```python
from build123d import *

# Parameters (mm, degrees)
SKETCH1_W           = 1000
SKETCH1_H           = 141
SKETCH1_H_2         = 170
SKETCH1_H_3         = 32
BOSS_EXTRUDE1_DEPTH = 40
SKETCH2_W           = 44
SKETCH2_H           = 44
BOSS_EXTRUDE2_DEPTH = 296
SKETCH3_W           = 44
SKETCH3_H           = 40
BOSS_EXTRUDE3_DEPTH = 100
SKETCH4_W           = 44
SKETCH4_H           = 44
BOSS_EXTRUDE4_DEPTH = 209


with BuildPart() as part:
    # Sketch1 → Boss-Extrude1 (new body)
    with BuildSketch(Plane(origin=(0, 0, 0), x_dir=(1, 0, 0), z_dir=(0, 1, 0))):
        Polygon((-500, 236), (-500, 345), (-540, 345), (-540, -345), (-500, -345), (-500, -283), (500, -283), (500, -345), (540, -345), (540, 345), (500, 345), (500, 236), align=None)
        with Locations((0, -168.5)):
            Rectangle(SKETCH1_W, SKETCH1_H, mode=Mode.SUBTRACT)
        with Locations((0, 31)):
            Rectangle(SKETCH1_W, SKETCH1_H_2, mode=Mode.SUBTRACT)
        with Locations((0, 176)):
            Rectangle(SKETCH1_W, SKETCH1_H_3, mode=Mode.SUBTRACT)
    extrude(amount=BOSS_EXTRUDE1_DEPTH)

    # Sketch2 → Boss-Extrude2 (add)
    with BuildSketch(Plane(origin=(0, 40, 0), x_dir=(1, 0, 0), z_dir=(0, 1, 0))):
        with Locations((-123, 214)):
            Rectangle(SKETCH2_W, SKETCH2_H)
        with Locations((123, 214)):
            Rectangle(SKETCH2_W, SKETCH2_H)
        with Locations((-123, 138)):
            Rectangle(SKETCH2_W, SKETCH2_H)
        with Locations((123, 138)):
            Rectangle(SKETCH2_W, SKETCH2_H)
    extrude(amount=BOSS_EXTRUDE2_DEPTH)

    # Sketch3 → Boss-Extrude3 (add)
    with BuildSketch(Plane.XY.offset(-116)):
        with Locations((-123, 20)):
            Rectangle(SKETCH3_W, SKETCH3_H)
        with Locations((123, 20)):
            Rectangle(SKETCH3_W, SKETCH3_H)
    extrude(amount=BOSS_EXTRUDE3_DEPTH)

    # Sketch4 → Boss-Extrude4 (add)
    with BuildSketch(Plane(origin=(-101, 0, 0), x_dir=(0, 0, -1), z_dir=(1, 0, 0))):
        with Locations((138, 210)):
            Rectangle(SKETCH4_W, SKETCH4_H)
        with Locations((214, 210)):
            Rectangle(SKETCH4_W, SKETCH4_H)
    extrude(amount=BOSS_EXTRUDE4_DEPTH)


solid = part.part
```
The model under review builds one solid part; all positions refer to its coordinate system, in mm. A direction names the side the tool comes from. Round coordinates to 2 decimals unless told otherwise and drop trailing zeros. Write each loop counter-clockwise with the first axis right and the second up, starting at its lowest first coordinate (ties: lowest second). Pieces come first, ordered by that corner, then holes. Notation, with made-up numbers: (13.25, 25) - (69.25, 25) arc R30 cw to (69.25, 52) - close; hole circle Ø9 at (-14, -38). An arc over 180 degrees is marked (long way). Use one line per item in the form item = value.
Q1. Consider section C-C (y = 164). State the section outline as (x, z) points.
Answer key:
outline = (-145, -236) - (-101, -236) - (-101, -192) - (-145, -192) - close; (-145, -160) - (-101, -160) - (-101, -116) - (-145, -116) - close; (101, -236) - (145, -236) - (145, -192) - (101, -192) - close; (101, -160) - (145, -160) - (145, -116) - (101, -116) - close
Q2. Tool access review of faces 1 (the flat face through (101, 113, -138)), 2 (the flat face through (145, 186, -214)), 3 (the flat face through (500, 20, 314)), 4 (the flat face through (-7, 20, 98)): name each direction out of +Z, -Z, +X, -X, +Y, -Y from which nothing blocks a thin tool from reaching the whole face with its end or side.
Answer key:
face_1 = +Z, -Z
face_2 = +Z, -Z, +X, +Y
face_3 = +Z, +Y, -Y
face_4 = +Y, -Y
Q3. Consider section D-D (x = -82.5). State the section outline as (y, z) points, and give its area (3 significant figures).
Answer key:
outline = (0, -236) - (40, -236) - (40, -192) - (0, -192) - close; (0, -160) - (40, -160) - (40, -116) - (0, -116) - close; (0, 54) - (40, 54) - (40, 98) - (0, 98) - close; (0, 239) - (40, 239) - (40, 283) - (0, 283) - close; (188, -236) - (232, -236) - (232, -192) - (188, -192) - close; (188, -160) - (232, -160) - (232, -116) - (188, -116) - close
area = 10,900 mm2
Q4. Draft analysis for pull direction X (two halves, no side actions). For faces 5 (the flat face through (-520, 20, -345)), 6 (the flat face through (-1, 188, -214)), 7 (the flat face through (540, 20, 5)), state which applies: +X half, -X half, draft (parallel to the pull), parting line (faces both ways), or undercut.
Answer key:
face_5 = draft
face_6 = undercut
face_7 = +X half
Q5. For line 1 (Y direction, x = 24.5, z = -140); line 2 (Z direction, x = -388, y = 29); line 3 (Z direction, x = -105.5, y = 124), list the stretches that pass through material, from the lowest coordinate up. Write a range as [from, to].
Answer key:
line_1 = [0, 40], [188, 232]
line_2 = [-236, -192], [-160, -116], [54, 98], [239, 283]
line_3 = [-236, -192], [-160, -116]
Q6. Insertion check: pin 1 Ø12 at (x, y) = (290.5, 16.5) entering from +Z; pin 2 Ø13 at (y, z) = (291, -135.5) entering from +X; pin 3 Ø13 at (x, z) = (-115.5, -65.5) entering from +Y. Each pin has a flat end and moves straight along its axis. Give the tip position at first contact, or say it passes through.
Answer key:
pin_1 = 283
pin_2 = 145
pin_3 = 40
Q7. Consider section A-A (z = 117). State the section outline as (x, y) points.
Answer key:
outline = (-540, 0) - (-500, 0) - (-500, 40) - (-540, 40) - close; (500, 0) - (540, 0) - (540, 40) - (500, 40) - close
Q8. Consider section B-B (x = 208). State the section outline as (y, z) points.
Answer key:
outline = (0, -236) - (40, -236) - (40, -192) - (0, -192) - close; (0, -160) - (40, -160) - (40, -116) - (0, -116) - close; (0, 54) - (40, 54) - (40, 98) - (0, 98) - close; (0, 239) - (40, 239) - (40, 283) - (0, 283) - close
